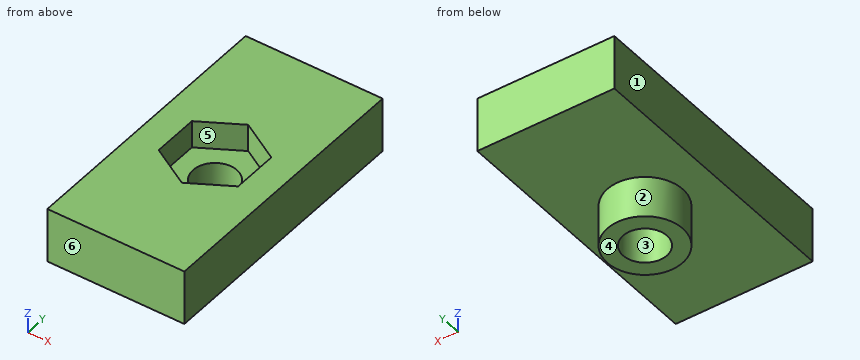
from build123d import *

# Parameters (mm, degrees)
SKETCH006_R   = 2.75
SKETCH006_R_2 = 1.6
PAD005_DEPTH  = 3
SKETCH008_R   = 3.5
SKETCH008_R_2 = 1.6
PAD006_DEPTH  = 2
SKETCH007_W   = 10
SKETCH007_H   = 20
PAD007_DEPTH  = 4


with BuildPart() as part:
    # Sketch006 → Pad005 (new body)
    with BuildSketch(Plane.XY):
        Circle(SKETCH006_R)
        Circle(SKETCH006_R_2, mode=Mode.SUBTRACT)
    extrude(amount=-PAD005_DEPTH)

    # Sketch008 → Pad006 (join)
    with BuildSketch(Plane.XY):
        Circle(SKETCH008_R)
        Circle(SKETCH008_R_2, mode=Mode.SUBTRACT)
    extrude(amount=PAD006_DEPTH)

    # Sketch007 → Pad007 (join)
    with BuildSketch(Plane.XY):
        Rectangle(SKETCH007_W, SKETCH007_H)
        Polygon((0, -3.348632), (2.9, -1.674316), (2.9, 1.674316), (0, 3.348632), (-2.9, 1.674316), (-2.9, -1.674316), align=None, mode=Mode.SUBTRACT)
    extrude(amount=PAD007_DEPTH)


solid = part.part
Check sheet for the modelled part. Datum: model origin and axes. Units: mm. Face numbers are marked on the shaded views. A direction names the side the tool comes from. Give positions to 0.01 mm unless a question says otherwise; leave off trailing zeros. Write each loop counter-clockwise with the first axis right and the second up, starting at its lowest first coordinate (ties: lowest second). Pieces come first, ordered by that corner, then holes. Notation, with made-up numbers: (-38, -14.75) -> (-28, -14.75) arc R22 ccw to (-28, -3.75) -> close; hole circle Ø5 at (-5.5, 84). An arc over 180 degrees is marked (long way). Use one line per item in the form item = value. Start each with the question number.
1. Thickness scan on line 1 along Y through (x, z) = (0, -0.85); line 2 along X through (y, z) = (1.25, 3); line 3 along Y through (x, z) = (0, 0.8). Record the ranges inside material, lowest first. Write a range as from..to.
2. Mould release check, pull along X, two halves, no side actions. Record for the marked faces 1, 2, 3 and 4: pulls with the +X half, pulls with the -X half, needs draft (parallel to the pull), parting line crosses it, or undercut.
3. Section check B-B (z = 2.5). Record the cut outline in (x, y).
4. Section check A-A (y = 0). Record the cut outline in (x, z).
5. Access from +Z, -Z, +X, -X, +Y, -Y to the whole of each face (thin tool, end or side, straight path). Record for the marked faces 5 and 6.
6. Section check C-C (x = 1.25). Record the cut outline in (y, z).
7. Section check D-D (x = -4). Record the cut outline in (y, z), and give its area (3 significant figures).
Conclusion:
q1.line_1 = -2.75..-1.6, 1.6..2.75
q1.line_2 = -5..-2.9, 2.9..5
q1.line_3 = -10..-1.6, 1.6..10
q2.face_1 = pulls with the -X half
q2.face_2 = parting line crosses it
q2.face_3 = undercut
q2.face_4 = needs draft
q3.outline = (-5, -10) -> (5, -10) -> (5, 10) -> (-5, 10) -> close; hole (-2.9, -1.67) -> (0, -3.35) -> (2.9, -1.67) -> (2.9, 1.67) -> (0, 3.35) -> (-2.9, 1.67) -> close
q4.outline = (-5, 0) -> (-2.75, 0) -> (-2.75, -3) -> (-1.6, -3) -> (-1.6, 2) -> (-2.9, 2) -> (-2.9, 4) -> (-5, 4) -> close; (1.6, -3) -> (2.75, -3) -> (2.75, 0) -> (5, 0) -> (5, 4) -> (2.9, 4) -> (2.9, 2) -> (1.6, 2) -> close
q5.face_5 = +Z
q5.face_6 = +Z, -Z, +X, -X, -Y
q6.outline = (-10, 0) -> (-2.45, 0) -> (-2.45, -3) -> (-1, -3) -> (-1, 2) -> (-2.63, 2) -> (-2.63, 4) -> (-10, 4) -> close; (1, -3) -> (2.45, -3) -> (2.45, 0) -> (10, 0) -> (10, 4) -> (2.63, 4) -> (2.63, 2) -> (1, 2) -> close
q7.outline = (-10, 0) -> (10, 0) -> (10, 4) -> (-10, 4) -> close
q7.area = 80.0 mm²
